The model under review builds one solid part; all positions refer to its coordinate system, in mm. A direction names the side the tool comes from. Round coordinates to 2 decimals unless told otherwise and drop trailing zeros. Write each loop counter-clockwise with the first axis right and the second up, starting at its lowest first coordinate (ties: lowest second). Pieces come first, ordered by that corner, then holes. Notation, with made-up numbers: (-33, 20.25) -> (-17, 20.25) arc R17 ccw to (-17, 31.25) -> close; hole circle Ø6 at (55.5, 35.5). An arc over 180 degrees is marked (long way). Return JSON: item names as keys, results as strings. Group by question number.
1. Take a section at A-A, the plane x = -8. Write out the cut boundary in (y, z).
2. Clearance check with flat-ended pins moving along their axes: P1, Ø3, axis at y = -8, z = 22, coming from the +X side; P2, Ø3, axis at y = 7.5, z = 12.5, coming from the +X side; P3, Ø6, axis at x = -30.5, y = 12.5, coming from the -Z side; P4, Ø10, axis at x = 24.5, y = 12, coming from the -Z side. State where each tip first meets the part, or that it passes through.
3. For line 1 along Z through (x, y) = (-30, -17); line 2 along Y through (x, z) = (-32.5, 12.5); line 3 along X through (y, z) = (-28, 14), list the stretches that pass through material, from the lowest coordinate up. Write a range as from..to.
4. Take a section at B-B, the plane z = 5. Write out the cut boundary in (x, y), then the cut area to 3 significant figures.
5. Tool access review of faces 1 (the flat face through (22.86, -7.6, 9.86)), 2 (the flat face through (-15, 27.173, 11)): name each direction out of +Z, -Z, +X, -X, +Y, -Y from which nothing blocks a thin tool from reaching the whole face with its end or side.
from build123d import *

# Parameters (mm, degrees)
F1_DEPTH = 25
F2_T     = -2.5
F3_R     = 5


with BuildPart() as f1:
    # F0 (on Top) → F1 (new body)
    with BuildSketch(Plane.XY):
        Polygon((12.2111159576, 29.6730460864), (-37.7888840424, 29.6730460864), (-37.7888840424, -40.3269539136), (32.2111159576, -40.3269539136), align=None)
    extrude(amount=F1_DEPTH)

    # F2
    f2_openings = [f1.faces().sort_by_distance(p)[0] for p in [
        (-37.788884, -5.326954, 12.5),
        (-7.511106, -7.271398, 0),
        (-2.788884, -40.326954, 12.5),
    ]]
    offset(amount=F2_T, openings=f2_openings)

    # F3
    f3_edges = [f1.edges().sort_by_distance(p)[0] for p in [
        (12.211116, 29.673046, 12.5),
        (10.325362, 27.173046, 11.25),
        (-12.788884, 29.673046, 25),
        (22.211116, -5.326954, 25),
        (-37.788884, 29.673046, 12.5),
    ]]
    fillet(f3_edges, radius=F3_R)


solid = f1.part
Output:
{
 "1": {"outline": "(-40.33, 22.5) -> (27.17, 22.5) -> (27.17, 0) -> (29.67, 0) -> (29.67, 20) arc R5 ccw to (24.67, 25) -> (-40.33, 25) -> close"},
 "2": {"P1": "stops at x = 23.19", "P2": "stops at x = 18.97", "P3": "stops at z = 22.5", "P4": "passes through"},
 "3": {"line 1": "z = 22.5..25", "line 2": "y = 27.17..29.67", "line 3": "x = 26.09..28.69"},
 "4": {"outline": "(-37.12, 27.17) -> (6.55, 27.17) arc R5 cw to (11.36, 23.55) -> (29.61, -40.33) -> (32.21, -40.33) -> (13.25, 26.05) arc R5 ccw to (8.44, 29.67) -> (-32.79, 29.67) arc R5 ccw to start", "area": "297 mm^2"},
 "5": {"face 1": "+Z, -Z, +X, +Y", "face 2": "-Z, -X, -Y"}
}
